```python
from build123d import *

# Parameters (mm, degrees)
SKETCH_1_W      = 40
SKETCH_1_H      = 40
EXTRUDE_1_DEPTH = 4
SKETCH_2_R      = 8
SKETCH_2_R_2    = 5
EXTRUDE_2_DEPTH = 12
FILLET_1_R      = 20


with BuildPart() as part:
    # Эскиз1 → Вытянуть1 (new body)
    with BuildSketch(Plane(origin=(0, 0, 0), x_dir=(1, 0, 0), z_dir=(0, 1, 0))):
        with Locations((20, 20)):
            Rectangle(SKETCH_1_W, SKETCH_1_H)
    extrude(amount=EXTRUDE_1_DEPTH)

    # Эскиз2 → Вытянуть2 (add)
    with BuildSketch(Plane(origin=(0, 4, 0), x_dir=(1, 0, 0), z_dir=(0, 1, 0))):
        with Locations(Location((20, 20, 0), (0, 0, 90))):
            Circle(SKETCH_2_R)
        with Locations(Location((20, 20, 0), (0, 0, 270))):
            Circle(SKETCH_2_R_2, mode=Mode.SUBTRACT)
    extrude(amount=EXTRUDE_2_DEPTH)

    # Скругление1
    fillet_1_edges = [part.edges().sort_by_distance(p)[0] for p in [
        (40, 2, 0),
        (0, 2, 0),
        (0, 2, -40),
        (40, 2, -40),
    ]]
    fillet(fillet_1_edges, radius=FILLET_1_R - 0.0001)  # a hair under: the kernel refuses the full size


solid = part.part
```
Here's how the part is built. I have some questions about the finished solid (model axes, mm). A direction names the side the tool comes from. Give positions to 0.01 mm unless a question says otherwise; leave off trailing zeros. Loops run counter-clockwise (first coordinate to the right, second up) from the corner with the lowest first, then second, coordinate; pieces in that order, holes last. Notation, with made-up numbers: M 78.25,42.5 L 87.25,42.5 A21 ccw 87.25,67.5 Z; hole C 26.25,-29.5 d10. An arc over 180 degrees is marked long. Put each result on its own line as item: value. Start each with the question number.
(1) Will these pins go through, and if not, where does the flat tip stop? pin 1 Ø8 at (x, z) = (20, -20) entering from +Y; pin 2 Ø4 at (y, z) = (4.5, -25) entering from -X; pin 3 Ø3 at (x, y) = (14, 11.5) entering from +Z.
(2) I want a section at D-D on x = 16.5. Please give me the cut outline in (y, z), then the cut area to 3 significant figures.
(3) I need wall thicknesses on line 1 along X through (y, z) = (12.5, -20); line 2 along Y through (x, z) = (15.5, -33); line 3 along X through (y, z) = (6.5, -23). Which ranges of each line are inside material? Lowest first, please. Write a range as [from, to].
(4) For faces 1 (the cylindrical face through (24.868, 9.916, -13.651)), 2 (the flat face through (25.2, 16, -19.9)), which set-ups out of +Z, -Z, +X, -X, +Y, -Y let a thin tool reach every point of the face, with its end or its side?
(5) I want a section at A-A on y = 11. Please give me the cut outline in (x, z), then the cut area to 3 significant figures.
(6) If we mould it in two halves opening along Z, with no side actions, what happens to faces 3 (the cylindrical face through (5.703, 2.028, -33.986)), 4 (the flat face through (20, 0, -20)), 5 (the flat face through (20, 4, -20))? For each: +Z half, -Z half, draft (parallel to the pull), parting line (faces both ways), or undercut.
(7) I want a section at C-C on x = 20.5. Please give me the cut outline in (y, z), then the cut area to 3 significant figures.
Answer block:
1. pin 1: y = 4
1. pin 2: x = 0.24
1. pin 3: z = -13.39
2. outline: M 0,-39.69 L 4,-39.69 L 4,-27.19 L 16,-27.19 L 16,-23.57 L 4,-23.57 L 4,-16.43 L 16,-16.43 L 16,-12.81 L 4,-12.81 L 4,-0.31 L 0,-0.31 Z
2. area: 244 mm^2
3. line 1: [12, 15], [25, 28]
3. line 2: [0, 4]
3. line 3: [12.58, 16], [24, 27.42]
4. face 1: +Y
4. face 2: +Z, -Z, +X, -X, +Y
5. outline: C 20,-20 d16; hole C 20,-20 d10
5. area: 123 mm^2
6. face 3: -Z half
6. face 4: draft
6. face 5: undercut
7. outline: M 0,-39.99 L 4,-39.99 L 4,-27.98 L 16,-27.98 L 16,-24.97 L 4,-24.97 L 4,-15.03 L 16,-15.03 L 16,-12.02 L 4,-12.02 L 4,-0.01 L 0,-0.01 Z
7. area: 232 mm^2
